Here's how the part is built. I have some questions about the finished solid (model axes, mm). Face numbers are marked on the shaded views. A direction names the side the tool comes from. Round coordinates to 2 decimals unless told otherwise and drop trailing zeros. Loops run counter-clockwise (first coordinate to the right, second up) from the corner with the lowest first, then second, coordinate; pieces in that order, holes last. Notation, with made-up numbers: M 84,-34 L 106,-34 A20 cw 106,-23 Z; hole C 36.5,87.25 d9. An arc over 180 degrees is marked long. Put each result on its own line as item: value. Start each with the question number.
```python
from build123d import *

# Parameters (mm, degrees)
SKETCH1_W           = 50
SKETCH1_H           = 15
SKETCH1_R           = 2
BOSS_EXTRUDE1_DEPTH = 3
SKETCH2_W           = 50
SKETCH2_H           = 3
BOSS_EXTRUDE2_DEPTH = 18
SKETCH3_R           = 2
CUT_EXTRUDE1_DEPTH  = 3


with BuildPart() as part:
    # Sketch1 → Boss-Extrude1 (new body)
    with BuildSketch(Plane(origin=(0, 0, 0), x_dir=(1, 0, 0), z_dir=(0, 1, 0))):
        Rectangle(SKETCH1_W, SKETCH1_H)
        with Locations(Location((0, -2.5, 0), (0, 0, 270))):
            Circle(SKETCH1_R, mode=Mode.SUBTRACT)
    extrude(amount=BOSS_EXTRUDE1_DEPTH)

    # Sketch2 → Boss-Extrude2 (add)
    with BuildSketch(Plane.XZ):
        with Locations((0, -9)):
            Rectangle(SKETCH2_W, SKETCH2_H)
    extrude(amount=-BOSS_EXTRUDE2_DEPTH)

    # Sketch3 → Cut-Extrude1 (cut)
    with BuildSketch(Plane.XY.offset(-7.5)):
        with Locations((-10, 10.5)):
            Circle(SKETCH3_R)
        with Locations(Location((10, 10.5, 0), (0, 0, 180))):
            Circle(SKETCH3_R)
    extrude(amount=-CUT_EXTRUDE1_DEPTH, mode=Mode.SUBTRACT)


solid = part.part
```
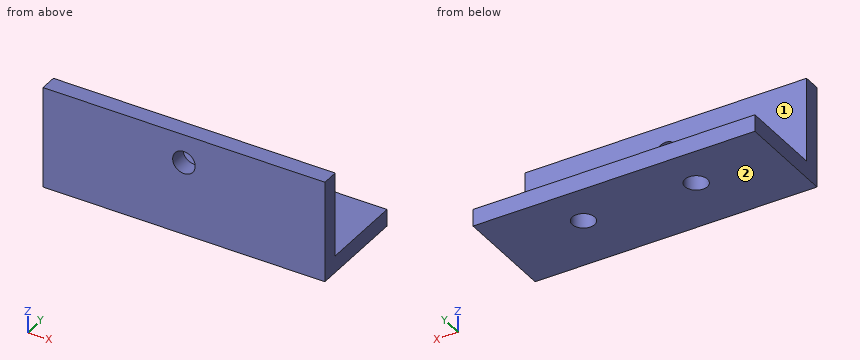
1) On a 3-axis mill with a long thin cutter (end or side, diameter ignored), from which of +Z, -Z, +X, -X, +Y, -Y can I reach the whole of each face in a straight line? I mean the marked faces 1 and 2. Say none if no direction works.
2) Suppose I cut it at D-D (z = 1). Write out the boundary of the cut face in (x, y).
3) Suppose I cut it at B-B (y = 10.5). Write out the boundary of the cut face in (x, z), plus the area to 3 significant figures.
4) Suppose I cut it at A-A (x = 0). Write out the boundary of the cut face in (y, z), plus the area to 3 significant figures.
5) Suppose I cut it at C-C (z = -8.25). Write out the boundary of the cut face in (x, y).
6) I'm going to push flat-ended pins straight in: P1, Ø5, axis at y = 10.5, z = -4.5, coming from the +X side; P2, Ø3, axis at x = -1, z = -4, coming from the +Y side; P3, Ø1, axis at x = -8, z = -8.5, coming from the -Y side; P4, Ø7.5, axis at x = -11.5, y = 13, coming from the +Z side. Where does each tip first touch, or does it pass through?
7) If I drill on probe 1 along X at (y, z) = (2.05, 2.5); probe 2 along Y at (x, z) = (-14.5, 1.75); probe 3 along Z at (x, y) = (8, 4.25), over which ranges is the centre line in solid material (lowest first)? Write a range as from..to.
Results are:
1. face 1: +Z, +X, -X, +Y
1. face 2: -Z, +X, -X, +Y, -Y
2. outline: M -25,0 L -1.32,0 L -1.32,3 L -25,3 Z; M 1.32,0 L 25,0 L 25,3 L 1.32,3 Z
3. outline: M -25,-10.5 L -12,-10.5 L -12,-7.5 L -25,-7.5 Z; M -8,-10.5 L 8,-10.5 L 8,-7.5 L -8,-7.5 Z; M 12,-10.5 L 25,-10.5 L 25,-7.5 L 12,-7.5 Z
3. area: 126 mm²
4. outline: M 0,-10.5 L 18,-10.5 L 18,-7.5 L 3,-7.5 L 3,0.5 L 0,0.5 Z; M 0,4.5 L 3,4.5 L 3,7.5 L 0,7.5 Z
4. area: 87.0 mm²
5. outline: M -25,0 L 25,0 L 25,18 L -25,18 Z; hole C -10,10.5 d4; hole C 10,10.5 d4
6. P1: through
6. P2: y = 3
6. P3: y = 0
6. P4: z = -7.5
7. probe 1: -25..-2, 2..25
7. probe 2: 0..3
7. probe 3: -10.5..-7.5
